Part model, mm, in its own coordinate system. Coordinates: 2 decimals unless noted, no trailing zeros. Order: outer loops, then holes, each group sorted by start corner. A loop starts at its lowest first (then second) coordinate and runs counter-clockwise, first axis right, second up.
1) Pin check, flat tips, straight feed: pin 1 Ø3 at (x, y) = (122.62, -129.51) entering from -Z; pin 2 Ø3 at (x, y) = (145.96, -87.07) entering from -Z. Stop position of each tip, or through.
2) Cut at B-B (x = 202.5). List the corners of the cut face in (y, z).
3) Cut at A-A (z = 2.3). Give the number of separate pieces and of enclosed holes in the cut face, and give its area (3 significant figures).
4) Wall check: L1, parallel to X at y = -81, z = 2; L2, parallel to X at y = -92.5, z = 1.95; L3, parallel to X at y = -141, z = 1.8. Give the ranges that are in metal, low to high.
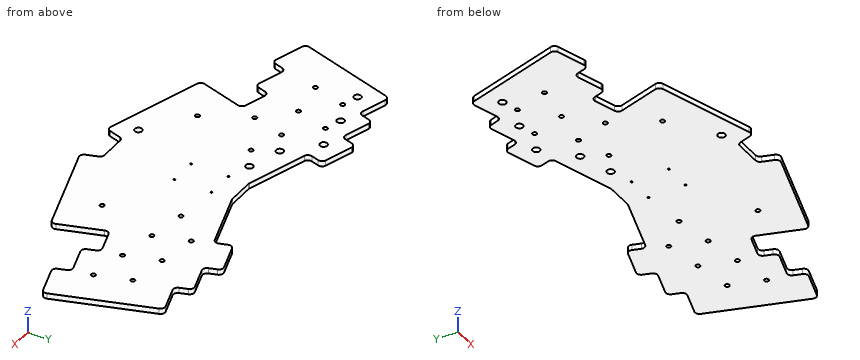
```python
from build123d import *

# Parameters (mm, degrees)
SKETCH1_R           = 1.190623
SKETCH1_R_2         = 1.190627
SKETCH1_R_3         = 1.190626
SKETCH1_R_4         = 1.190625
SKETCH1_R_5         = 1.190624
SKETCH1_R_6         = 1.190628
SKETCH1_R_7         = 1.9939
SKETCH1_R_8         = 0.5
BOSS_EXTRUDE1_DEPTH = 3


with BuildPart() as part:
    # Sketch1 → Boss-Extrude1 (new body)
    with BuildSketch(Plane.XY):
        with BuildLine():
            Line((104.968827, -55.794314), (103.615653, -60.086042))
            ThreePointArc((103.615653, -60.086042), (102.385728566, -61.551801144), (100.479593, -61.718568))
            Line((100.479593, -61.718568), (87.127552, -57.508685))
            ThreePointArc((87.127552, -57.508685), (85.221400275, -57.675416583), (83.9915, -59.141213))
            Line((83.9915, -59.141213), (82.638323, -63.432941))
            ThreePointArc((82.638323, -63.432941), (81.408394852, -64.898690118), (79.502266, -65.065473))
            Line((79.502266, -65.065473), (66.150224, -60.855587))
            ThreePointArc((66.150224, -60.855587), (64.244088242, -61.02234775), (63.014174, -62.488115))
            Line((63.014174, -62.488115), (46.776059, -113.988833))
            ThreePointArc((46.776059, -113.988833), (46.942822186, -115.894968516), (48.408585, -117.124888))
            Line((48.408585, -117.124888), (63.668055, -121.936181))
            ThreePointArc((63.668055, -121.936181), (65.574204538, -121.769435597), (66.804115, -120.303649))
            Line((66.804115, -120.303649), (68.157287, -116.011926))
            ThreePointArc((68.157287, -116.011926), (69.387211331, -114.546165389), (71.293348, -114.379399))
            Line((71.293348, -114.379399), (84.645384, -118.589282))
            ThreePointArc((84.645384, -118.589282), (86.551538999, -118.422552795), (87.78144, -116.956753))
            Line((87.78144, -116.956753), (89.134615, -112.665026))
            ThreePointArc((89.134615, -112.665026), (90.364542844, -111.19927904), (92.27067, -111.032498))
            Line((92.27067, -111.032498), (103.715276, -114.640965))
            ThreePointArc((103.715276, -114.640965), (105.181030723, -115.870890231), (105.347808, -117.777022))
            Line((105.347808, -117.777022), (98.281218, -140.189373))
            ThreePointArc((98.281218, -140.189373), (98.447984756, -142.095508452), (99.913747, -143.325429))
            Line((99.913747, -143.325429), (151.414462, -159.563543))
            ThreePointArc((151.414462, -159.563543), (153.320596182, -159.396771864), (154.550517, -157.931011))
            Line((154.550517, -157.931011), (156.499763, -151.748809))
            ThreePointArc((156.499763, -151.748809), (157.405773888, -150.484456349), (158.88405, -150.000573))
            Line((158.88405, -150.000573), (173.000221, -150.000576))
            ThreePointArc((173.000221, -150.000576), (174.478488224, -150.484472097), (175.384512, -151.74881))
            Line((175.384512, -151.74881), (177.333756, -157.931011))
            ThreePointArc((177.333756, -157.931011), (178.563666363, -159.396793874), (180.469813, -159.563539))
            Line((180.469813, -159.563539), (231.970529, -143.32543))
            ThreePointArc((231.970529, -143.32543), (233.436289923, -142.095506386), (233.603057, -140.18937))
            Line((233.603057, -140.18937), (226.536464, -117.777022))
            ThreePointArc((226.536464, -117.777022), (226.703215942, -115.870876032), (228.168999, -114.640966))
            Line((228.168999, -114.640966), (239.613602, -111.032497))
            ThreePointArc((239.613602, -111.032497), (241.519721203, -111.199292709), (242.749655, -112.665026))
            Line((242.749655, -112.665026), (244.102833, -116.956749))
            ThreePointArc((244.102833, -116.956749), (245.33275051, -118.422517183), (247.238889, -118.589279))
            Line((247.238889, -118.589279), (260.590925, -114.379399))
            ThreePointArc((260.590925, -114.379399), (262.497073777, -114.546144678), (263.726987, -116.011928))
            Line((263.726987, -116.011928), (265.080159, -120.303654))
            ThreePointArc((265.080159, -120.303654), (266.310073195, -121.769434184), (268.21622, -121.936182))
            Line((268.21622, -121.936182), (283.47569, -117.124888))
            ThreePointArc((283.47569, -117.124888), (284.94147585, -115.894978684), (285.108216, -113.98883))
            Line((285.108216, -113.98883), (268.870102, -62.488115))
            ThreePointArc((268.870102, -62.488115), (267.640181911, -61.022352077), (265.734046, -60.855588))
            Line((265.734046, -60.855588), (252.382012, -65.065468))
            ThreePointArc((252.382012, -65.065468), (250.475863383, -64.898725926), (249.245954, -63.43294))
            Line((249.245954, -63.43294), (247.892776, -59.141216))
            ThreePointArc((247.892776, -59.141216), (246.662867771, -57.67543136), (244.756721, -57.508688))
            Line((244.756721, -57.508688), (231.40468, -61.718568))
            ThreePointArc((231.40468, -61.718568), (229.498544633, -61.551806932), (228.268627, -60.086043))
            Line((228.268627, -60.086043), (226.915449, -55.794313))
            ThreePointArc((226.915449, -55.794313), (225.685509928, -54.328581771), (223.779389, -54.161785))
            Line((223.779389, -54.161785), (208.519923, -58.973078))
            ThreePointArc((208.519923, -58.973078), (207.054132, -60.202983526), (206.887395, -62.109134))
            Line((206.887395, -62.109134), (208.240572, -66.400862))
            ThreePointArc((208.240572, -66.400862), (208.073804347, -68.306999096), (206.608041, -69.536921))
            Line((206.608041, -69.536921), (173.90813, -79.84716))
            ThreePointArc((173.90813, -79.84716), (173.536675423, -79.933776781), (173.156367, -79.962871))
            Line((173.156367, -79.962871), (158.727909, -79.962872))
            ThreePointArc((158.727909, -79.962872), (158.347599344, -79.933772207), (157.976142, -79.84716))
            Line((157.976142, -79.84716), (125.276233, -69.536916))
            ThreePointArc((125.276233, -69.536916), (123.81048285, -68.30698987), (123.643706, -66.400861))
            Line((123.643706, -66.400861), (124.996881, -62.109136))
            ThreePointArc((124.996881, -62.109136), (124.830112452, -60.203001632), (123.364354, -58.973078))
            Line((123.364354, -58.973078), (108.104881, -54.161784))
            ThreePointArc((108.104881, -54.161784), (106.198732394, -54.328524877), (104.968827, -55.794314))
        make_face()
        with Locations((260.771527, -103.312897)):
            Circle(SKETCH1_R, mode=Mode.SUBTRACT)
        with Locations((255.058117, -85.19229)):
            Circle(SKETCH1_R_2, mode=Mode.SUBTRACT)
        with Locations((239.794198, -99.965999)):
            Circle(SKETCH1_R_3, mode=Mode.SUBTRACT)
        with Locations((234.080792, -81.845377)):
            Circle(SKETCH1_R_4, mode=Mode.SUBTRACT)
        with Locations((218.816871, -96.619099)):
            Circle(SKETCH1_R_5, mode=Mode.SUBTRACT)
        with Locations((213.103463, -78.498475)):
            Circle(SKETCH1_R_4, mode=Mode.SUBTRACT)
        with Locations((197.839541, -93.272199)):
            Circle(SKETCH1_R_6, mode=Mode.SUBTRACT)
        with Locations((209.266366, -129.513445)):
            Circle(SKETCH1_R_5, mode=Mode.SUBTRACT)
        with Locations((122.617905, -129.51344)):
            Circle(SKETCH1_R_2, mode=Mode.SUBTRACT)
        with Locations((134.044729, -93.272199)):
            Circle(SKETCH1_R_4, mode=Mode.SUBTRACT)
        with Locations((110.210695, -105.679413)):
            Circle(SKETCH1_R_3, mode=Mode.SUBTRACT)
        with Locations((115.924107, -87.558799)):
            Circle(SKETCH1_R_4, mode=Mode.SUBTRACT)
        with Locations((100.660188, -72.785066)):
            Circle(SKETCH1_R_4, mode=Mode.SUBTRACT)
        with Locations((94.946783, -90.905689)):
            Circle(SKETCH1_R_4, mode=Mode.SUBTRACT)
        with Locations((73.969454, -94.252592)):
            Circle(SKETCH1_R_4, mode=Mode.SUBTRACT)
        with Locations((79.584014, -76.043701)):
            Circle(SKETCH1_R_2, mode=Mode.SUBTRACT)
        with Locations((146.942133, -147.143868)):
            Circle(SKETCH1_R_7, mode=Mode.SUBTRACT)
        with Locations((145.961745, -87.068589)):
            Circle(SKETCH1_R_7, mode=Mode.SUBTRACT)
        with Locations((127.841123, -81.355183)):
            Circle(SKETCH1_R_7, mode=Mode.SUBTRACT)
        with Locations((112.577207, -66.581459)):
            Circle(SKETCH1_R_7, mode=Mode.SUBTRACT)
        with Locations((91.599877, -69.928361)):
            Circle(SKETCH1_R_7, mode=Mode.SUBTRACT)
        with Locations((70.622553, -73.275262)):
            Circle(SKETCH1_R_7, mode=Mode.SUBTRACT)
        with Locations((158.322139, -111.478591)):
            Circle(SKETCH1_R_8, mode=Mode.SUBTRACT)
        with Locations((173.562139, -111.478591)):
            Circle(SKETCH1_R_8, mode=Mode.SUBTRACT)
        with Locations((173.562139, -91.158591)):
            Circle(SKETCH1_R_8, mode=Mode.SUBTRACT)
        with Locations((158.322139, -91.158591)):
            Circle(SKETCH1_R_8, mode=Mode.SUBTRACT)
    extrude(amount=BOSS_EXTRUDE1_DEPTH)


solid = part.part
```
Geometry check:
1. pin 1: stops at z = 0
1. pin 2: passes through
2. outline: (-152.62, 0) - (-70.83, 0) - (-70.83, 3) - (-152.62, 3) - close
3. separate pieces: 1
3. enclosed holes: 26
3. area: 15,700 mm2
4. L1: x = 57.18 to 125.88, 129.8 to 233.24, 234.92 to 274.71
4. L2: x = 53.55 to 133.14, 134.95 to 196.93, 198.75 to 278.33
4. L3: x = 98.17 to 233.72
